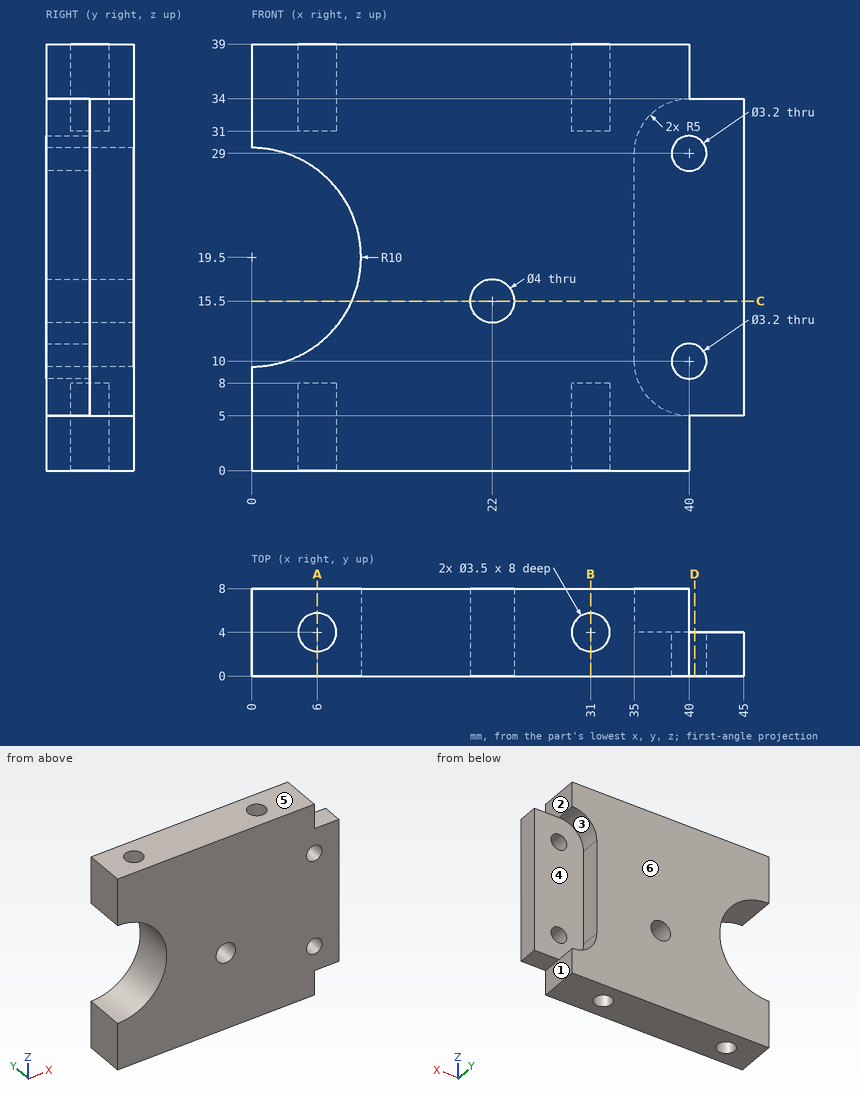
Design review of the part shown in the three views and the two pictorial views. Dimensions are in mm from the part's minimum x, y and z. A direction names the side the tool comes from. Round coordinates to 2 decimals unless told otherwise and drop trailing zeros. Write each loop counter-clockwise with the first axis right and the second up, starting at its lowest first coordinate (ties: lowest second). Pieces come first, ordered by that corner, then holes.
Item 1: Consider section D-D on x = 40.5. Give the boundary of the cut face in (y, z).
Item 2: Consider section A-A on x = 6. Give the boundary of the cut face in (y, z), and give its area (3 significant figures).
Item 3: Consider section C-C on z = 15.5. Give the boundary of the cut face in (x, y).
Item 4: For the marked faces 1, 2 and 3, list the 3-axis set-ups (+Z, -Z, +X, -X, +Y, -Y) from which the entire face can be reached by the end or side of a thin tool; tool diameter is ignored.
Item 5: For pin 1 Ø1.2 at (y, z) = (5.5, 23) entering from +X; pin 2 Ø4.5 at (x, y) = (6, 4) entering from +Z; pin 3 Ø3.5 at (x, z) = (40, 10) entering from +Y; pin 4 Ø1.2 at (x, y) = (41.5, 2.5) entering from -Z, all flat-tipped, find the tip position at first contact; note any pin that passes through.
Item 6: Wall thickness on L1, parallel to X at y = 5, z = 35; L2, parallel to Y at x = 6, z = 33; L3, parallel to Z at x = 21.5, y = 4.25: over which ranges is each line inside the solid? List them lowest first.
Item 7: Consider section B-B on x = 31. Give the boundary of the cut face in (y, z).
Item 8: Draft analysis for pull direction Z (two halves, no side actions). For the marked faces 4, 5 and 6, state which applies: released by +Z, released by -Z, zero draft, split by the parting line, or undercut.
Check values:
1. outline: (0, 5) - (4, 5) - (4, 8.48) - (0, 8.48) - close; (0, 11.52) - (4, 11.52) - (4, 27.48) - (0, 27.48) - close; (0, 30.52) - (4, 30.52) - (4, 34) - (0, 34) - close
2. outline: (0, 0) - (2.25, 0) - (2.25, 8) - (5.75, 8) - (5.75, 0) - (8, 0) - (8, 11.5) - (0, 11.5) - close; (0, 27.5) - (8, 27.5) - (8, 39) - (5.75, 39) - (5.75, 31) - (2.25, 31) - (2.25, 39) - (0, 39) - close
2. area: 128 mm2
3. outline: (9.17, 0) - (20, 0) - (20, 8) - (9.17, 8) - close; (24, 0) - (45, 0) - (45, 4) - (35, 4) - (35, 8) - (24, 8) - close
4. face 1: -Z, +X, +Y, -Y
4. face 2: +Z, +X, +Y, -Y
4. face 3: +X, +Y
5. pin 1: stops at x = 35
5. pin 2: stops at z = 39
5. pin 3: stops at y = 4
5. pin 4: stops at z = 5
6. L1: x = 0 to 4.56, 7.44 to 29.56, 32.44 to 40
6. L2: y = 0 to 2.25, 5.75 to 8
6. L3: z = 0 to 13.56, 17.44 to 39
7. outline: (0, 0) - (2.25, 0) - (2.25, 8) - (5.75, 8) - (5.75, 0) - (8, 0) - (8, 39) - (5.75, 39) - (5.75, 31) - (2.25, 31) - (2.25, 39) - (0, 39) - close
8. face 4: undercut
8. face 5: released by +Z
8. face 6: zero draft
